```python
from build123d import *

# Parameters (mm, degrees)
SKETCH3_R                = 7.408333333
BOSS_EXTRUDE1_DEPTH      = 7.62
CUT_EXTRUDE1_START       = -8.62
CUT_EXTRUDE1_DEPTH       = 9.62
FILLET1_R                = 0.355076163
CIRPATTERN1_COUNT        = 12
FILLET1_OF_CIRPATTERN1_R = 0.355076163
SCALE1_SCALE             = 2.5
SKETCH10_R               = 27.94
BOSS_EXTRUDE4_DEPTH      = 10.16
SKETCH11_R               = 5.08
CUT_EXTRUDE5_DEPTH       = 30.21
CUT_EXTRUDE6_DEPTH       = 5.08
SKETCH13_R               = 1.5875
CUT_EXTRUDE12_DEPTH      = 25.1300001
SKETCH16_R               = 2.74955
CUT_EXTRUDE13_DEPTH      = 3.81
SKETCH18_R               = 5.08
BOSS_EXTRUDE5_DEPTH      = 24.13
SKETCH19_R               = 2.794
CUT_EXTRUDE14_DEPTH      = 22.86
SKETCH20_R               = 1.5875
CUT_EXTRUDE15_DEPTH      = 7.62
SKETCH21_R               = 26.202104712
GEAR_CUT_EXTRUDE_DEPTH   = 19.05
SKETCH22_R               = 1.651
CUT_EXTRUDE17_DEPTH      = 10.16
SKETCH23_R               = 2.921
CUT_EXTRUDE18_DEPTH      = 3.048


with BuildPart() as part:
    # Sketch3 → Boss-Extrude1 (new body)
    with BuildSketch(Plane.XY):
        Circle(SKETCH3_R)
    extrude(amount=-BOSS_EXTRUDE1_DEPTH)

    # Sketch4 → Cut-Extrude1 (cut)
    with BuildSketch(Plane.XY.offset(CUT_EXTRUDE1_START)):
        with BuildLine():
            Line((4.993301754, 0.581811335), (5.926950078, 0.690598508))
            add(Edge.make_bspline(
                [(5.926950078, 0.690598508), (5.929318191, 0.690911872), (5.935944647, 0.691904892), (5.948407954, 0.694232443), (5.96863478, 0.69866684), (5.994230847, 0.70524939), (6.027084964, 0.714822349), (6.065467787, 0.727462413), (6.107282331, 0.74277265), (6.152345854, 0.760950457), (6.196898763, 0.780422108), (6.240942495, 0.801081108), (6.284441008, 0.822769247), (6.336662498, 0.8503395), (6.398612769, 0.885198626), (6.469984516, 0.92853373), (6.54965538, 0.980716028), (6.629400976, 1.037091207), (6.706647925, 1.095172788), (6.78320647, 1.156800213), (6.856219389, 1.218511327), (6.930432721, 1.285554849), (6.998115798, 1.348944008), (7.07205666, 1.423150182), (7.131183599, 1.483972917), (7.190627906, 1.549410219), (7.219315962, 1.581641114), (7.233873511, 1.598273068)],
                knots=[0, 0, 0, 0, 0, 0.005376749, 0.015083688, 0.02853182, 0.046610139, 0.064854849, 0.092110525, 0.119476176, 0.146842496, 0.174208854, 0.201574956, 0.228941013, 0.256307345, 0.307035032, 0.361767352, 0.416499661, 0.471231937, 0.525964282, 0.580696615, 0.635428982, 0.690161387, 0.744893688, 0.799626082, 0.854358408, 0.909090915, 0.909090915, 0.909090915, 0.909090915, 0.909090915], degree=4))
            ThreePointArc((7.233873511, 1.598273068), (7.408333333, 0), (7.233873511, -1.598273068))
            add(Edge.make_bspline(
                [(5.926950078, -0.690598508), (5.929318191, -0.690911872), (5.935944647, -0.691904892), (5.948407954, -0.694232443), (5.96863478, -0.69866684), (5.994230847, -0.70524939), (6.027084964, -0.714822349), (6.065467787, -0.727462413), (6.107282331, -0.74277265), (6.152345854, -0.760950457), (6.196898763, -0.780422108), (6.240942495, -0.801081108), (6.284441008, -0.822769247), (6.336662498, -0.8503395), (6.398612769, -0.885198626), (6.469984516, -0.92853373), (6.54965538, -0.980716028), (6.629400976, -1.037091207), (6.706647925, -1.095172788), (6.78320647, -1.156800213), (6.856219389, -1.218511327), (6.930432721, -1.285554849), (6.998115798, -1.348944008), (7.07205666, -1.423150182), (7.131183599, -1.483972917), (7.190627906, -1.549410219), (7.219315962, -1.581641114), (7.233873511, -1.598273068)],
                knots=[0, 0, 0, 0, 0, 0.005376749, 0.015083688, 0.02853182, 0.046610139, 0.064854849, 0.092110525, 0.119476176, 0.146842496, 0.174208854, 0.201574956, 0.228941013, 0.256307345, 0.307035032, 0.361767352, 0.416499661, 0.471231937, 0.525964282, 0.580696615, 0.635428982, 0.690161387, 0.744893688, 0.799626082, 0.854358408, 0.909090915, 0.909090915, 0.909090915, 0.909090915, 0.909090915], degree=4))
            Line((5.926950078, -0.690598508), (4.993301754, -0.581811335))
            ThreePointArc((4.993301754, -0.581811335), (5.027083333, 0), (4.993301754, 0.581811335))
        make_face()
    cut_extrude1 = extrude(amount=CUT_EXTRUDE1_DEPTH, mode=Mode.SUBTRACT)

    # Fillet1
    fillet1_edges = [part.edges().sort_by_distance(p)[0] for p in [
        (4.993301754, -0.581811335, -3.81),
        (4.993301754, 0.581811335, -3.81),
    ]]
    fillet(fillet1_edges, radius=FILLET1_R)

    # CirPattern1: Cut-Extrude1 ×12 about axis
    cirpattern1_axis = Axis((0, 0, 6.35), (0, 0, -1))
    for i in range(1, CIRPATTERN1_COUNT):
        add(cut_extrude1.rotate(cirpattern1_axis, i * 360 / CIRPATTERN1_COUNT), mode=Mode.SUBTRACT)

    # Fillet1 of CirPattern1
    fillet1_of_cirpattern1_edges = [part.edges().sort_by_distance(p)[0] for p in [
        (4.0334205, -3.000514274, -3.81),
        (4.615231836, -1.99278748, -3.81),
        (1.99278748, -4.615231836, -3.81),
        (3.000514274, -4.0334205, -3.81),
        (-0.581811335, -4.993301754, -3.81),
        (0.581811335, -4.993301754, -3.81),
        (-3.000514274, -4.0334205, -3.81),
        (-1.99278748, -4.615231836, -3.81),
        (-4.615231836, -1.99278748, -3.81),
        (-4.0334205, -3.000514274, -3.81),
        (-4.993301754, 0.581811335, -3.81),
        (-4.993301754, -0.581811335, -3.81),
        (-4.0334205, 3.000514274, -3.81),
        (-4.615231836, 1.99278748, -3.81),
        (-1.99278748, 4.615231836, -3.81),
        (-3.000514274, 4.0334205, -3.81),
        (0.581811335, 4.993301754, -3.81),
        (-0.581811335, 4.993301754, -3.81),
        (3.000514274, 4.0334205, -3.81),
        (1.99278748, 4.615231836, -3.81),
        (4.615231836, 1.99278748, -3.81),
        (4.0334205, 3.000514274, -3.81),
    ]]
    fillet(fillet1_of_cirpattern1_edges, radius=FILLET1_OF_CIRPATTERN1_R)


with BuildPart() as part_1:
    # Scale1: scaled about (0, 0, 0)
    add(part.part.scale(SCALE1_SCALE))

    # Sketch10 → Boss-Extrude4 (add)
    with BuildSketch(Plane.XY):
        Circle(SKETCH10_R)
    extrude(amount=BOSS_EXTRUDE4_DEPTH)

    # Sketch11 → Cut-Extrude5 (cut, through all)
    with BuildSketch(Plane(origin=(0, 0, -19.05), x_dir=(-1, 0, 0), z_dir=(0, 0, -1))):
        Circle(SKETCH11_R)
    extrude(amount=-CUT_EXTRUDE5_DEPTH, mode=Mode.SUBTRACT)

    # Sketch12 → Cut-Extrude6 (cut)
    with BuildSketch(Plane.XY.offset(10.16)):
        with BuildLine():
            Line((-10.080312495, -3.81), (-28.438556916, -3.81))
            Line((-28.438556916, -3.81), (-28.438556916, 3.81))
            Line((-28.438556916, 3.81), (-10.080312495, 3.81))
            ThreePointArc((-10.080312495, 3.81), (-7.386235659, 4.302142678), (-5.040156248, 5.715))
            ThreePointArc((-5.040156248, 5.715), (7.62, 0), (-5.040156248, -5.715))
            ThreePointArc((-5.040156248, -5.715), (-7.386235659, -4.302142678), (-10.080312495, -3.81))
        make_face()
    extrude(amount=-CUT_EXTRUDE6_DEPTH, mode=Mode.SUBTRACT)

    # Sketch13 → Cut-Extrude12 (cut, through all)
    with BuildSketch(Plane.XY.offset(5.08)):
        with Locations((-19.812, 0)):
            Circle(SKETCH13_R)
    extrude(amount=-CUT_EXTRUDE12_DEPTH, mode=Mode.SUBTRACT)

    # Sketch16 → Cut-Extrude13 (cut)
    with BuildSketch(Plane(origin=(0, 0, 0), x_dir=(-1, 0, 0), z_dir=(0, 0, -1))):
        with Locations((19.812, 0)):
            Circle(SKETCH16_R)
    extrude(amount=-CUT_EXTRUDE13_DEPTH, mode=Mode.SUBTRACT)

    # Sketch18 → Boss-Extrude5 (add)
    with BuildSketch(Plane(origin=(0, 0, -19.05), x_dir=(-1, 0, 0), z_dir=(0, 0, -1))):
        Circle(SKETCH18_R)
    extrude(amount=-BOSS_EXTRUDE5_DEPTH)

    # Sketch19 → Cut-Extrude14 (cut)
    with BuildSketch(Plane(origin=(0, 0, -19.05), x_dir=(-1, 0, 0), z_dir=(0, 0, -1))):
        Circle(SKETCH19_R)
    extrude(amount=-CUT_EXTRUDE14_DEPTH, mode=Mode.SUBTRACT)

    # Sketch20 → Cut-Extrude15 (cut)
    with BuildSketch(Plane(origin=(0, 0, 3.81), x_dir=(-1, 0, 0), z_dir=(0, 0, -1))):
        Circle(SKETCH20_R)
    extrude(amount=-CUT_EXTRUDE15_DEPTH, mode=Mode.SUBTRACT)

    # Sketch21 → Gear Cut Extrude (cut)
    with BuildSketch(Plane(origin=(0, 0, -19.05), x_dir=(-1, 0, 0), z_dir=(0, 0, -1))):
        Circle(SKETCH21_R)
    extrude(amount=-GEAR_CUT_EXTRUDE_DEPTH, mode=Mode.SUBTRACT)

    # Sketch22 → Cut-Extrude17 (cut)
    with BuildSketch(Plane.XY.offset(10.16)):
        with Locations((0, 12.7)):
            Circle(SKETCH22_R)
        with Locations((0, -12.7)):
            Circle(SKETCH22_R)
    extrude(amount=-CUT_EXTRUDE17_DEPTH, mode=Mode.SUBTRACT)

    # Sketch23 → Cut-Extrude18 (cut)
    with BuildSketch(Plane.XY.offset(10.16)):
        with Locations((0, -12.7)):
            Circle(SKETCH23_R)
        with Locations((0, 12.7)):
            Circle(SKETCH23_R)
    extrude(amount=-CUT_EXTRUDE18_DEPTH, mode=Mode.SUBTRACT)


solid = part_1.part
```
For this review, take the finished solid that the model builds, in its own axes (mm). A direction names the side the tool comes from. Give positions to 0.01 mm unless a question says otherwise; leave off trailing zeros. Write each loop counter-clockwise with the first axis right and the second up, starting at its lowest first coordinate (ties: lowest second). Pieces come first, ordered by that corner, then holes. Notation, with made-up numbers: M 11,-23.75 L 21,-23.75 A11 cw 21,-12.75 Z; hole C 37.25,39.5 d6. An arc over 180 degrees is marked long. Answer as a JSON object with one key per item and string values. Group by question number.
Item 1: Draft analysis for pull direction X (two halves, no side actions). For faces 4 (the flat face through (1.3, -14, 7.112)), 5 (the flat face through (-19, -3.81, 8)), 6 (the cylindrical face through (26.65, 8.39, 5.01)), state which applies: +X half, -X half, draft (parallel to the pull), parting line (faces both ways), or undercut.
Item 2: Consider section D-D on y = -12. Write out the cut boundary in (x, z).
Item 3: Consider section A-A on x = 0. Count the separate pieces of the cut face and the enclosed holes in it, plus the area to 3 significant figures.
Item 4: Consider section B-B on y = 0. Write out the cut boundary in (x, z), plus the area to 3 significant figures.
Item 5: For pin 1 Ø4 at (x, y) = (0, 0) entering from -Z; pin 2 Ø3 at (x, y) = (-19.812, 0) entering from +Z; pin 3 Ø4.5 at (x, y) = (0, 12.7) entering from +Z; pin 4 Ø1.5 at (x, z) = (-23, 9) entering from +Y, all flat-tipped, find the tip position at first contact; note any pin that passes through.
Item 6: Tool access review of faces 1 (the flat face through (-10, 0, 5.08)), 2 (the cylindrical face through (2.217, -1.7, 1.878)), 3 (the flat face through (-19, 3.81, 8)): name each direction out of +Z, -Z, +X, -X, +Y, -Y from which nothing blocks a thin tool from reaching the whole face with its end or side.
Item 7: For probe 1 along Y at (x, z) = (0, 8.35); probe 2 along Y at (x, z) = (0, 3.75); probe 3 along X at (y, z) = (-0.5, 5), list the stretches that pass through material, from the lowest coordinate up. Write a range as [from, to].
Item 8: Consider section C-C on z = 9.5. Write out the cut boundary in (x, y) (3 decimals), plus the area to 3 significant figures.
Check result:
{
 "1": {"face 4": "undercut", "face 5": "draft", "face 6": "parting line"},
 "2": {"outline": "M -25.23,0 L -1.5,0 L -1.5,7.11 L -2.84,7.11 L -2.84,10.16 L -25.23,10.16 Z; M 1.5,0 L 25.23,0 L 25.23,10.16 L 2.84,10.16 L 2.84,7.11 L 1.5,7.11 Z"},
 "3": {"separate pieces": "4", "enclosed holes": "0", "area": "382 mm^2"},
 "4": {"outline": "M -27.94,0 L -22.56,0 L -22.56,3.81 L -21.4,3.81 L -21.4,5.08 L -27.94,5.08 Z; M -18.22,3.81 L -17.06,3.81 L -17.06,0 L -2.79,0 L -2.79,3.81 L -1.59,3.81 L -1.59,5.08 L -18.22,5.08 Z; M 1.59,3.81 L 2.79,3.81 L 2.79,0 L 27.94,0 L 27.94,10.16 L 7.62,10.16 L 7.62,5.08 L 1.59,5.08 Z", "area": "337 mm^2"},
 "5": {"pin 1": "stops at z = 3.81", "pin 2": "passes through", "pin 3": "stops at z = 7.11", "pin 4": "stops at y = 16.9"},
 "6": {"face 1": "+Z", "face 2": "-Z", "face 3": "+Z, -X"},
 "7": {"probe 1": "y = [-27.94, -15.62], [-9.78, -7.62], [7.62, 9.78], [15.62, 27.94]", "probe 2": "y = [-27.94, -14.35], [-11.05, -2.79], [2.79, 11.05], [14.35, 27.94]", "probe 3": "x = [-27.94, -21.32], [-18.31, -1.51], [1.51, 27.94]"},
 "8": {"outline": "M -27.679,-3.81 A27.94 ccw long -27.679,3.81 L -10.08,3.81 A7.62 ccw -5.04,5.715 A7.62 cw long -5.04,-5.715 A7.62 ccw -10.08,-3.81 Z; hole C 0,-12.7 d5.842; hole C 0,12.7 d5.842", "area": "2,060 mm^2"}
}
